Build history of the part. All positions in model axes, mm. A direction names the side the tool comes from. Give positions to 0.01 mm unless a question says otherwise; leave off trailing zeros. Loops run counter-clockwise (first coordinate to the right, second up) from the corner with the lowest first, then second, coordinate; pieces in that order, holes last. Notation, with made-up numbers: (8.25, 1.5) -> (58.25, 1.5) arc R20 ccw to (58.25, 5.5) -> close; hole circle Ø9 at (19.5, -40). An arc over 180 degrees is marked (long way). Answer as a JSON object with one key per item and string values. Group by question number.
Q1. Wall check: probe 1 along Z at (x, y) = (-3, 10.5); probe 2 along X at (y, z) = (0, -2.5); probe 3 along Z at (x, y) = (-8, 11.25). Give the ranges that are in metal, low to high. Write a range as from..to.
Q2. Band-saw the part on C-C, the plane x = -11.25. Write the cut outline in (y, z), plus the area to 3 significant figures.
Q3. Tool access for faces 4 (the flat face through (-1, -4, 2.5)), 5 (the flat face through (0, 15, -5)): list every direction of +Z, -Z, +X, -X, +Y, -Y with a clear straight run to the whole face (end or side of a thin tool).
Q4. Band-saw the part on A-A, the plane y = 0. Write the cut outline in (x, z).
Q5. Two-plate mould, pull along X, no slides. Class faces 1 (the cylindrical face through (6.396, 0.676, 3.732)), 2 (the flat face through (0, -15, -5)), 3 (the cylindrical face through (-2.17, -9.76, 2.46)): pulls with the +X half, pulls with the -X half, needs draft (parallel to the pull), parting line crosses it, or undercut.
Q6. Drop flat-ended pins along their axis: pin 1 (2 mm diameter, centred on x = -3, y = 4.5, fed in from +Z); pin 2 (1.5 mm diameter, centred on x = -4, z = -2, fed in from +Y). Give the stop position or say it passes through.
Q7. Band-saw the part on B-B, the plane x = 4.25. Write the cut outline in (y, z), plus the area to 3 significant figures.
from build123d import *

# Parameters (mm, degrees)
CYLINDER157_R     = 2.25
CYLINDER157_DEPTH = 8
CYLINDER156_R     = 1
CYLINDER156_DEPTH = 18
CYLINDER147_R     = 1
CYLINDER147_DEPTH = 1
ARRAY_COUNT       = 3
CYLINDER153_R     = 10
CYLINDER153_DEPTH = 5
BOX_W             = 30
BOX_H             = 30
BOX_DEPTH         = 2
CYLINDER202_R     = 12
CYLINDER202_DEPTH = 6


with BuildPart() as sealsubtraction:
    # Cylinder157 → Cylinder157 (new body)
    with BuildSketch(Plane.XY.offset(2.5)):
        Circle(CYLINDER157_R)
    extrude(amount=CYLINDER157_DEPTH)


with BuildPart() as bottomwireoutlet:
    # Cylinder156 → Cylinder156 (new body)
    with BuildSketch(Plane.XY.offset(-8)):
        Circle(CYLINDER156_R)
    extrude(amount=CYLINDER156_DEPTH)


with BuildPart() as sealarray:
    # Cylinder147 → Cylinder147 (new body)
    with BuildSketch(Plane.XY.offset(4.5)):
        Circle(CYLINDER147_R)
    extrude(amount=CYLINDER147_DEPTH)

    # Fusion: union SealSubtraction, BottomWireOutlet
    add(sealsubtraction.part)
    add(bottomwireoutlet.part)


with BuildPart() as sealarray_1:
    # Fusion placement: moved
    add(sealarray.part.moved(Location((4.25, 0, 0))))

    # Array: SealArray ×3 about axis
    array_axis = Axis((0, 0, 0), (0, 0, 1))


with BuildPart() as sealarray_2:
    add(sealarray_1.part)
    for i in range(1, ARRAY_COUNT):
        add(sealarray_1.part.rotate(array_axis, i * 360 / ARRAY_COUNT))


with BuildPart() as body:
    # Cylinder153 → Cylinder153 (new body)
    with BuildSketch(Plane.XY):
        Circle(CYLINDER153_R)
    extrude(amount=CYLINDER153_DEPTH)


with BuildPart() as cube:
    # Box → Box (new body)
    with BuildSketch(Plane(origin=(-15, -15, -6), x_dir=(1, 0, 0), z_dir=(0, 0, 1))):
        with Locations((15, 15)):
            Rectangle(BOX_W, BOX_H)
    extrude(amount=BOX_DEPTH)


with BuildPart() as cut:
    # Cylinder202 → Cylinder202 (new body)
    with BuildSketch(Plane.XY.offset(-6)):
        Circle(CYLINDER202_R)
    extrude(amount=CYLINDER202_DEPTH)

    # Fusion012: union Body, Cube
    add(body.part)
    add(cube.part)

    # Cut: cut SealArray
    add(sealarray_2.part, mode=Mode.SUBTRACT)


solid = cut.part
Worked answers:
{
 "1": {"probe 1": "-6..0", "probe 2": "-12..3.25, 5.25..12", "probe 3": "-6..-4"},
 "2": {"outline": "(-15, -6) -> (15, -6) -> (15, -4) -> (4.18, -4) -> (4.18, 0) -> (-4.18, 0) -> (-4.18, -4) -> (-15, -4) -> close", "area": "93.4 mm2"},
 "3": {"face 4": "+Z", "face 5": "+Z, -Z, +X, -X, +Y"},
 "4": {"outline": "(-15, -6) -> (3.25, -6) -> (3.25, 2.5) -> (2, 2.5) -> (2, 5) -> (-10, 5) -> (-10, 0) -> (-12, 0) -> (-12, -4) -> (-15, -4) -> close; (5.25, -6) -> (15, -6) -> (15, -4) -> (12, -4) -> (12, 0) -> (10, 0) -> (10, 5) -> (6.5, 5) -> (6.5, 2.5) -> (5.25, 2.5) -> close"},
 "5": {"face 1": "undercut", "face 2": "needs draft", "face 3": "parting line crosses it"},
 "6": {"pin 1": "z = 2.5", "pin 2": "y = 11.55"},
 "7": {"outline": "(-15, -6) -> (-1, -6) -> (-1, 2.5) -> (-2.25, 2.5) -> (-2.25, 5) -> (-9.05, 5) -> (-9.05, 0) -> (-11.22, 0) -> (-11.22, -4) -> (-15, -4) -> close; (1, -6) -> (15, -6) -> (15, -4) -> (11.22, -4) -> (11.22, 0) -> (9.05, 0) -> (9.05, 5) -> (2.25, 5) -> (2.25, 2.5) -> (1, 2.5) -> close", "area": "212 mm2"}
}
